```python
from build123d import *

# Parameters (mm, degrees)
SKETCH1_R                  = 4
BOSS_EXTRUDE1_DEPTH        = 2.032
BOSS_EXTRUDE3_DEPTH        = 10.668
SKETCH12_R                 = 1.36525
CUT_EXTRUDE2_DEPTH         = 4
CUT_EXTRUDE3_DEPTH         = 6
CUT_EXTRUDE3_DEPTH_BACK    = 1
SKETCH14_R                 = 1.35255
FILLET1_R                  = 10
FLATTEN_BENDS1_START       = 2
FLATTEN_BENDS1_DEPTH       = 10.668
FLATTEN_BENDS1_START_2     = -0.032
FLATTEN_BENDS1_2_OUTLINE_R = 1.36525
FLATTEN_BENDS1_2_DEPTH     = 2.032
PROCESS_BENDS1_START       = -9.067864684
PROCESS_BENDS1_OUTLINE_W   = 29
PROCESS_BENDS1_OUTLINE_H   = 2.032
PROCESS_BENDS1_DEPTH       = 9.398
PROCESS_BENDS1_START_2     = 0.620942425
PROCESS_BENDS1_2_OUTLINE_W = 29
PROCESS_BENDS1_2_OUTLINE_H = 10.668
PROCESS_BENDS1_2_OUTLINE_R = 1.36525
PROCESS_BENDS1_2_DEPTH     = 1.71084748
PROCESS_BENDS1_START_3     = 0.330135316
PROCESS_BENDS1_3_OUTLINE_W = 29
PROCESS_BENDS1_3_OUTLINE_H = 2.032
PROCESS_BENDS1_3_DEPTH     = 0.184274429
PROCESS_BENDS1_START_4     = 0.299789905
PROCESS_BENDS1_4_OUTLINE_W = 29
PROCESS_BENDS1_4_OUTLINE_H = 10.668
PROCESS_BENDS1_4_OUTLINE_R = 1.36525
PROCESS_BENDS1_4_DEPTH     = 3.302
PROCESS_BENDS1_START_5     = -6.292093187
PROCESS_BENDS1_5_DEPTH     = 29


with BuildPart() as part:
    # Sketch1 → Boss-Extrude1 (new body)
    with BuildSketch(Plane(origin=(0, 2, 0), x_dir=(1, 0, 0), z_dir=(0, 1, 0))):
        with BuildLine():
            Line((16.268898369, 15.844931419), (-4.237198285, -4.661165235))
            Line((-4.237198285, -4.661165235), (7.60163648, -16.5))
            Line((7.60163648, -16.5), (48.167251499, -16.5))
            Line((48.167251499, -16.5), (66.344250399, -13.294904666))
            ThreePointArc((66.344250399, -13.294904666), (77.499939542, -0.040402458), (66.423785357, 13.280634945))
            ThreePointArc((66.423785357, 13.280634945), (42.528480772, 15.498562339), (18.613829789, 13.5))
            Line((18.613829789, 13.5), (16.268898369, 15.844931419))
        make_face()
        with Locations(Location((64, 0, 0), (0, 0, 90))):
            Circle(SKETCH1_R, mode=Mode.SUBTRACT)
    extrude(amount=-BOSS_EXTRUDE1_DEPTH)

    # Sketch5 → Boss-Extrude3 (add)
    with BuildSketch(Plane(origin=(0, 2, 0), x_dir=(1, 0, 0), z_dir=(0, 1, 0))):
        Polygon((16.268898369, 15.844931419), (-4.237198285, -4.661165235), (-2.800357306, -6.098006215), (17.705739349, 14.40809044), align=None)
    extrude(amount=BOSS_EXTRUDE3_DEPTH)

    # Sketch12 → Cut-Extrude2 (cut)
    with BuildSketch(Plane(origin=(0.211983475, 0, 0.211983475), x_dir=(-0.7071067811865475, 0, 0.7071067811865477), z_dir=(-0.7071067811865477, 0, -0.7071067811865475))):
        with Locations((-16.207906813, 7.968)):
            Circle(SKETCH12_R)
        with Locations((-0.207906813, 7.968)):
            Circle(SKETCH12_R)
    extrude(amount=-CUT_EXTRUDE2_DEPTH, mode=Mode.SUBTRACT)

    # Sketch14 → Cut-Extrude3 (cut, two sides: drawn at the far end of the back side and taken through both)
    with BuildSketch(Plane(origin=(0, 0, 0), x_dir=(1, 0, 0), z_dir=(0, 1, 0)).offset(-CUT_EXTRUDE3_DEPTH_BACK)):
        with Locations(Location((39.946755384, 11.867587507, 0), (0, 0, 270))):
            Circle(SKETCH14_R)
    extrude(amount=CUT_EXTRUDE3_DEPTH + CUT_EXTRUDE3_DEPTH_BACK, mode=Mode.SUBTRACT)

    # Fillet1
    fillet1_edges = [part.edges().sort_by_distance(p)[0] for p in [
        (7.60163648, 0.984, 16.5),
    ]]
    fillet(fillet1_edges, radius=FILLET1_R)

    # Flatten-Bends1: read off the stored shape, not the designer's step
    # Flatten-Bends1 outline → Flatten-Bends1 (cut)
    with BuildSketch(Plane(origin=(0, 0, 0), x_dir=(1, 0, 0), z_dir=(0, 1, 0)).offset(FLATTEN_BENDS1_START)):
        Polygon((17.705739349, 14.40809044), (16.290355815, 15.823473974), (16.268898369, 15.844931419), (-4.237198285, -4.661165235), (-2.800357306, -6.098006215), align=None)
    extrude(amount=FLATTEN_BENDS1_DEPTH, mode=Mode.SUBTRACT)

    # Flatten-Bends1 2 outline → Flatten-Bends1 2 (add)
    with BuildSketch(Plane(origin=(0, 0, 0), x_dir=(1, 0, 0), z_dir=(0, 1, 0)).offset(FLATTEN_BENDS1_START_2)):
        Polygon((-4.237198285, -4.661165235), (16.268898369, 15.844931419), (9.644966285, 22.468863503), (-10.861130369, 1.962766849), align=None)
        with Locations((-2.94153442, 3.235559055)):
            Circle(FLATTEN_BENDS1_2_OUTLINE_R, mode=Mode.SUBTRACT)
        with Locations((8.372174079, 14.549267554)):
            Circle(FLATTEN_BENDS1_2_OUTLINE_R, mode=Mode.SUBTRACT)
    extrude(amount=FLATTEN_BENDS1_2_DEPTH)

    # Process-Bends1: read off the stored shape, not the designer's step
    # Process-Bends1 outline → Process-Bends1 (cut)
    with BuildSketch(Plane(origin=(0, 0, 0), x_dir=(0.7071067811865474, 0, -0.7071067811865477), z_dir=(0.7071067811865476, 0, 0.7071067811865476)).offset(PROCESS_BENDS1_START)):
        with Locations((8.207906813, 0.984)):
            Rectangle(PROCESS_BENDS1_OUTLINE_W, PROCESS_BENDS1_OUTLINE_H)
    extrude(amount=PROCESS_BENDS1_DEPTH, mode=Mode.SUBTRACT)

    # Process-Bends1 2 outline → Process-Bends1 2 (add)
    with BuildSketch(Plane(origin=(0, 0, 0), x_dir=(0.7071067811865474, 0, -0.7071067811865477), z_dir=(0.7071067811865476, 0, 0.7071067811865476)).offset(PROCESS_BENDS1_START_2)):
        with Locations((8.207906813, 7.334)):
            Rectangle(PROCESS_BENDS1_2_OUTLINE_W, PROCESS_BENDS1_2_OUTLINE_H)
        with Locations((0.207906813, 7.968)):
            Circle(PROCESS_BENDS1_2_OUTLINE_R, mode=Mode.SUBTRACT)
        with Locations((16.207906813, 7.968)):
            Circle(PROCESS_BENDS1_2_OUTLINE_R, mode=Mode.SUBTRACT)
    extrude(amount=PROCESS_BENDS1_2_DEPTH)

    # Process-Bends1 3 outline → Process-Bends1 3 (cut)
    with BuildSketch(Plane(origin=(0, 0, 0), x_dir=(0.7071067811865474, 0, -0.7071067811865477), z_dir=(0.7071067811865476, 0, 0.7071067811865476)).offset(PROCESS_BENDS1_START_3)):
        with Locations((8.207906813, 0.984)):
            Rectangle(PROCESS_BENDS1_3_OUTLINE_W, PROCESS_BENDS1_3_OUTLINE_H)
    extrude(amount=PROCESS_BENDS1_3_DEPTH, mode=Mode.SUBTRACT)

    # Process-Bends1 4 outline → Process-Bends1 4 (add)
    with BuildSketch(Plane(origin=(0, 0, 0), x_dir=(0.7071067811865474, 0, -0.7071067811865477), z_dir=(0.7071067811865476, 0, 0.7071067811865476)).offset(PROCESS_BENDS1_START_4)):
        with Locations((8.207906813, 7.334)):
            Rectangle(PROCESS_BENDS1_4_OUTLINE_W, PROCESS_BENDS1_4_OUTLINE_H)
        with Locations((0.207906813, 7.968)):
            Circle(PROCESS_BENDS1_4_OUTLINE_R, mode=Mode.SUBTRACT)
        with Locations((16.207906813, 7.968)):
            Circle(PROCESS_BENDS1_4_OUTLINE_R, mode=Mode.SUBTRACT)
    extrude(amount=PROCESS_BENDS1_4_DEPTH)

    # Process-Bends1 5 outline → Process-Bends1 5 (cut)
    with BuildSketch(Plane(origin=(0, 0, 0), x_dir=(0.707106781186548, 0, 0.707106781186547), z_dir=(0.707106781186547, 0, -0.707106781186548)).offset(PROCESS_BENDS1_START_5)):
        with BuildLine():
            ThreePointArc((3.601789905, -2), (2.703764293, -2.371974388), (2.331789905, -3.27))
            Line((2.331789905, -3.27), (2.331789905, -12.668))
            Line((2.331789905, -12.668), (3.601789905, -12.668))
            Line((3.601789905, -12.668), (3.601789905, -2))
        make_face()
        with BuildLine():
            Line((0.299789905, -2), (0.299789905, -3.27))
            ThreePointArc((0.299789905, -3.27), (1.266923314, -0.935133409), (3.601789905, 0.032))
            Line((3.601789905, 0.032), (0.514409745, 0.032))
            Line((0.514409745, 0.032), (0.514409745, -2))
            Line((0.514409745, -2), (0.299789905, -2))
        make_face()
    extrude(amount=PROCESS_BENDS1_5_DEPTH, mode=Mode.SUBTRACT)


solid = part.part
```
Design review of the part built by this model. Coordinates are the model's own, in mm. A direction names the side the tool comes from. Coordinates: 2 decimals unless noted, no trailing zeros. Order: outer loops, then holes, each group sorted by start corner. A loop starts at its lowest first (then second) coordinate and runs counter-clockwise, first axis right, second up. Notation, with made-up numbers: (85, 18) - (129, 18) arc R23 cw to (129, 27) - close; hole circle Ø3 at (28.5, 89). An arc over 180 degrees is marked (long way). Answer in a Markdown table with one row per item.
(1) Consider section B-B on y = 10.5. State the section outline as (x, z) points, plus the area to 3 significant figures.
Checked values:
| item | result |
|---|---|
| outline | (-4.24, 4.66) - (16.27, -15.84) - (17.71, -14.41) - (-2.8, 6.1) - close |
| area | 58.9 mm^2 |
(2) Consider section C-C on z = 15.5. State the section outline as (x, y) points.
Checked values:
| item | result |
|---|---|
| outline | (7.38, -0.03) - (53.84, -0.03) - (53.84, 2) - (7.38, 2) - close |
(3) Clearance check with flat-ended pins moving along their axes: pin 1 (2 mm diameter, centred on x = 67.5, y = 1.5, fed in from -Z); pin 2 (1 mm diameter, centred on y = 6.5, z = -9.5, fed in from -X); pin 3 (12 mm diameter, centred on x = 22.5, z = 6.5, fed in from +Y). State where each tip first meets the part, or that it passes through.
Checked values:
| item | result |
|---|---|
| pin 1 | z = -13.27 |
| pin 2 | x = 9.42 |
| pin 3 | y = 2 |
(4) The part is to be moulded in two halves that separate along Y. For faces 1 (the cylindrical face through (0.94, 9.32, 0.9)), 2 (the flat face through (7, 12.668, -5)), 3 (the cylindrical face through (67.905, 0.998, 0.867)), say which applies: released by +Y, released by -Y, zero draft, split by the parting line, or undercut.
Checked values:
| item | result |
|---|---|
| face 1 | undercut |
| face 2 | released by +Y |
| face 3 | zero draft |
(5) For faces 4 (the flat face through (37, 2, 0)), 5 (the cylindrical face through (7.87, 0.97, 15.72)), list the 3-axis set-ups (+Z, -Z, +X, -X, +Y, -Y) from which the entire face can be reached by the end or side of a thin tool; tool diameter is ignored.
Checked values:
| item | result |
|---|---|
| face 4 | +Z, +X, +Y |
| face 5 | +Z, -X, +Y, -Y |
(6) Wall thickness on line 1 along Y through (x, z) = (34.5, 9.5); line 2 along Z through (x, y) = (64, 1.1); line 3 along X through (y, z) = (1.3, 0): over which ranges is each line inside the solid? List them lowest first. Write a range as from..to.
Checked values:
| item | result |
|---|---|
| line 1 | -0.03..2 |
| line 2 | -13.7..-4, 4..13.71 |
| line 3 | 1.35..60, 68..77.5 |
(7) Consider section A-A on x = 64. State the section outline as (y, z) points, plus the area to 3 significant figures.
Checked values:
| item | result |
|---|---|
| outline | (-0.03, -13.7) - (2, -13.7) - (2, -4) - (-0.03, -4) - close; (-0.03, 4) - (2, 4) - (2, 13.71) - (-0.03, 13.71) - close |
| area | 39.4 mm^2 |
